```python
from build123d import *

# Parameters (mm, degrees)
F2_R     = 4
F3_DEPTH = 9.2181856301


with BuildPart() as f1:
    # F0 (on Front) → F1 (revolve)
    with BuildSketch(Plane.XZ):
        Polygon((0, -35.3728421032), (0, 34.6271578968), (-30, 34.6271578968), (-13.8952266212, 11.6271578968), (-13.8952266212, 2.6271578968), (-29.5514642168, -26.3728421032), (-41.5514642168, -26.3728421032), (-41.5514642168, -17.3728421032), (-51.5514642168, -17.3728421032), (-45, -35.3728421032), align=None)
    revolve(axis=Axis((0, 0, -0.3728421032), (0, 0, -1)))

    # F2 (on face) → F3 (cut, through all)
    with BuildSketch(Plane(origin=(0, 0, -35.3728421032), x_dir=(1, 0, 0), z_dir=(0, 0, -1))):
        with Locations((-33.4342122078, 0)):
            Circle(F2_R)
        with Locations((-23.6415581758, -23.6415581758)):
            Circle(F2_R)
        with Locations((0, -33.4342122078)):
            Circle(F2_R)
        with Locations((23.6415581758, -23.6415581758)):
            Circle(F2_R)
        with Locations((33.4342122078, 0)):
            Circle(F2_R)
        with Locations((23.6415581758, 23.6415581758)):
            Circle(F2_R)
        with Locations((0, 33.4342122078)):
            Circle(F2_R)
        with Locations((-23.6415581758, 23.6415581758)):
            Circle(F2_R)
    extrude(amount=-F3_DEPTH, mode=Mode.SUBTRACT)


solid = f1.part
```
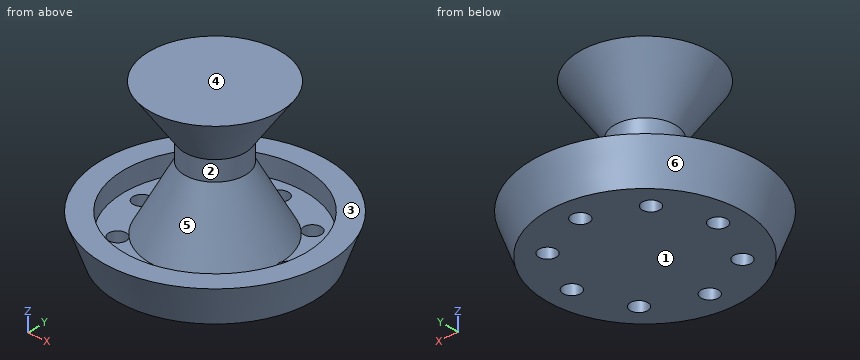
Verification items for the finished model (mm, model axes). Face numbers are marked on the shaded views. A direction names the side the tool comes from. Coordinates: 2 decimals unless noted, no trailing zeros. Order: outer loops, then holes, each group sorted by start corner. A loop starts at its lowest first (then second) coordinate and runs counter-clockwise, first axis right, second up. Notation, with made-up numbers: (81.25, -12) -> (86.25, -12) arc R9 cw to (86.25, -6) -> close; hole circle Ø7 at (14.5, 70.5). An arc over 180 degrees is marked (long way). Answer as CSV lines item,"result". Start each with the question number.
1) Release check for a two-part mould opening along Y. For the marked faces 4, 5 and 6 record: released by +Y, released by -Y, zero draft, split by the parting line, or undercut.
2) Gauge pin test, flat ends, axial feed: pin 1 Ø8 at (y, z) = (-19.5, 4.5) entering from +X; pin 2 Ø8 at (x, y) = (-8, 35.5) entering from +Z. Record the tip position at first contact, or that the pin passes through.
3) Cross-section at A-A, the plane z = -29.5. Give the number of separate pieces and of enclosed holes in the cut face, then the cut area to 3 significant figures.
4) Cross-section at D-D, the plane z = 13.5. Record the boundary of the cut face in (x, y).
5) Material ranges on L1, parallel to X at y = 0, z = -32; L2, parallel to X at y = 14.5, z = -22; L3, parallel to Z at x = -29, y = -23.5, recorded low to high. Write a range as [from, to].
6) Cross-section at C-C, the plane z = -12. Record the boundary of the cut face in (x, y).
7) Set-up check for the marked faces 1, 2 and 3: record each of +Z, -Z, +X, -X, +Y, -Y from which the full face is reachable in a straight line by a thin tool's end or side.
Conclusion:
1,face 4,"zero draft"
1,face 5,"undercut"
1,face 6,"split by the parting line"
2,pin 1,"passes through"
2,pin 2,"stops at z = -26.37"
3,separate pieces,"1"
3,enclosed holes,"8"
3,area,"6,580 mm²"
4,outline,"circle Ø30.41 at (0, 0)"
5,L1,"x = [-46.23, -37.43], [-29.43, 29.43], [37.43, 46.23]"
5,L2,"x = [-47.71, -38.94], [-23, 23], [38.94, 47.71]"
5,L3,"z = [-35.37, -26.37]"
6,outline,"circle Ø43.58 at (0, 0)"
7,face 1,"-Z, +X, -X, +Y, -Y"
7,face 2,"none"
7,face 3,"+Z"
